from build123d import *

# Parameters (mm, degrees)
F1_DEPTH = 18


with BuildPart() as f1:
    # F0 (on Top) → F1 (new body)
    with BuildSketch(Plane.XY):
        with BuildLine():
            ThreePointArc((-700.46645, -50), (129.221957, 690.257151), (634.9435, -300))
            Line((634.9435, -300), (956.296227, -300))
            ThreePointArc((956.296227, -300), (126.965132, 994.174194), (-1000.998961, -50.035513))
            Line((-1000.998961, -50.035513), (-999.705072, -50))
            Line((-999.705072, -50), (-700.46645, -50))
        make_face()
    extrude(amount=F1_DEPTH)


solid = f1.part
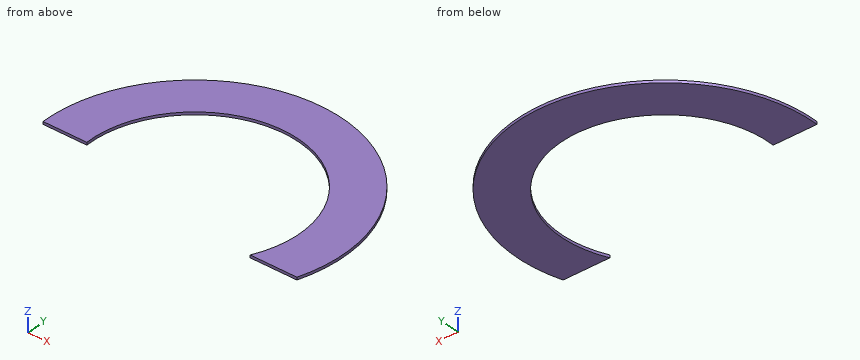
Can you work these out from the model? Positions are in its coordinate system, mm. Round coordinates to 2 decimals unless told otherwise and drop trailing zeros. Write each loop counter-clockwise with the first axis right and the second up, starting at its lowest first coordinate (ties: lowest second). Pieces come first, ordered by that corner, then holes. Notation, with made-up numbers: (-35.5, -36.75) - (0.5, -36.75) arc R19 ccw to (0.5, -31.75) - close; hole circle Ø8 at (40, 2). An arc over 180 degrees is marked (long way). Write each question's results on one line, items separated by ' | '. Start each with the question number.
1) Please list where these lines run through material, in increasing order: line 1 (X direction, y = 0, z = 5.5); line 2 (Y direction, x = 0, z = 5); line 3 (X direction, y = 39, z = 7.5).
2) Suppose I cut it at A-A (y = 0). List the corners of the cut face in (x, z) for me, and give its area (3 significant figures).
3) Suppose I cut it at D-D (y = 827.5). List the corners of the cut face in (x, z) for me, and give its area (3 significant figures).
4) For pin 1 Ø1 at (y, z) = (859, 8.5) entering from -X; pin 2 Ø2 at (y, z) = (699.5, 3) entering from +X; pin 3 Ø1 at (x, z) = (384.5, 13.5) entering from +Y, each with a flat end and sliding along its axis, tell me the tip position at first contact or that it passes through.
5) Suppose I cut it at C-C (x = 0). List the corners of the cut face in (y, z) for me, and give its area (3 significant figures).
6) Suppose I cut it at B-B (z = 6). List the corners of the cut face in (x, y) for me.
Here are the results:
1) line 1: x = -1002.25 to -702.25, 702.25 to 1002.25 | line 2: y = 702.25 to 1002.25 | line 3: x = -1001.49 to -701.16, 701.16 to 1001.49
2) outline: (-1002.25, 0) - (-702.25, 0) - (-702.25, 18) - (-1002.25, 18) - close; (702.25, 0) - (1002.25, 0) - (1002.25, 18) - (702.25, 18) - close | area: 10,800 mm2
3) outline: (-565.46, 0) - (565.46, 0) - (565.46, 18) - (-565.46, 18) - close | area: 20,400 mm2
4) pin 1: stops at x = -517.18 | pin 2: stops at x = 718.75 | pin 3: stops at y = 925.77
5) outline: (702.25, 0) - (1002.25, 0) - (1002.25, 18) - (702.25, 18) - close | area: 5,400 mm2
6) outline: (-1001, -50.04) - (-999.71, -50) - (-700.47, -50) arc R702.25 cw (long way) to (634.94, -300) - (956.3, -300) arc R1002.25 ccw (long way) to start
